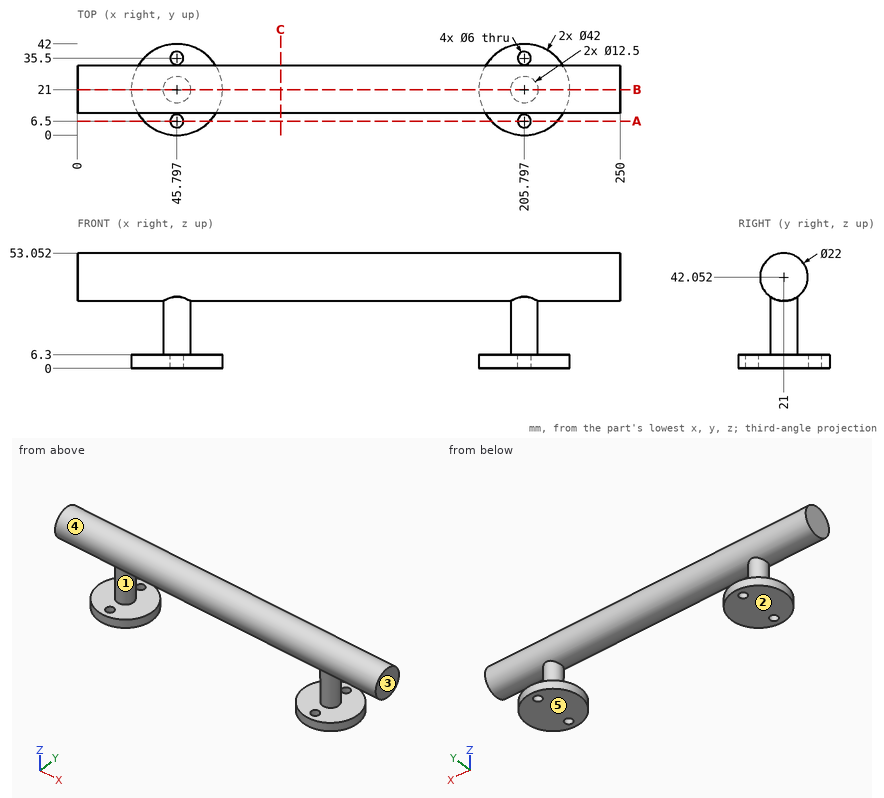
Geometry: see drawing. Coordinates: mm, zero at the bounding-box minimum. A direction names the side the tool comes from. Round coordinates to 2 decimals unless told otherwise and drop trailing zeros. Loops run counter-clockwise (first coordinate to the right, second up) from the corner with the lowest first, then second, coordinate; pieces in that order, holes last. Notation, with made-up numbers: (-25, -21) - (-1, -21) arc R18 ccw to (-1, -15) - close; hole circle Ø5 at (1, 27.5). An arc over 180 degrees is marked (long way). Write item = value, one per line. Start each with the question number.
(1) Set-up query: the marked faces 4 and 5. Return all of +Z, -Z, +X, -X, +Y, -Y with unobstructed straight access to the full face (end or side cutting, diameter ignored); none if empty.
(2) Section query A-A, the plane y = 6.5. Output: boundary loops of the cut face in (x, z).
(3) Section query B-B, the plane y = 21. Output: boundary loops of the cut face in (x, z).
(4) Pull-direction query (X, two-part tool) for the marked faces 1, 2 and 3; classes: +X half, -X half, draft (parallel to the pull), parting line (faces both ways), or undercut.
(5) Pin query (flat end, axial travel): pin 1 (4 mm diameter, centred on x = 204, y = 14, fed in from +Z); pin 2 (1 mm diameter, centred on x = 35.5, z = 36.5, fed in from +Y); pin 3 (5 mm diameter, centred on x = 80, z = 33, fed in from -Y) (1 decimal); pin 4 (8 mm diameter, centred on y = 14, z = 30.5, fed in from -X). Return the tip coordinate at first contact, or that it passes through.
(6) Section query C-C, the plane x = 93.5. Output: boundary loops of the cut face in (y, z), plus the area to 3 significant figures.
(7) Ray query, line 1 along X through (y, z) = (20.5, 22); line 2 along Y through (x, z) = (45, 3.5) (1 decimal); line 3 along Z through (x, y) = (56, 6). Return the intervals inside material, ascending. Write a range as from..to.
Conclusion:
q1.face_4 = none
q1.face_5 = -Z, +X, -X, +Y, -Y
q2.outline = (30.61, 0) - (42.8, 0) - (42.8, 6.3) - (30.61, 6.3) - close; (48.8, 0) - (60.99, 0) - (60.99, 6.3) - (48.8, 6.3) - close; (190.61, 0) - (202.8, 0) - (202.8, 6.3) - (190.61, 6.3) - close; (208.8, 0) - (220.99, 0) - (220.99, 6.3) - (208.8, 6.3) - close
q3.outline = (0, 31.05) - (39.55, 31.05) - (39.55, 6.3) - (24.8, 6.3) - (24.8, 0) - (66.8, 0) - (66.8, 6.3) - (52.05, 6.3) - (52.05, 31.05) - (199.55, 31.05) - (199.55, 6.3) - (184.8, 6.3) - (184.8, 0) - (226.8, 0) - (226.8, 6.3) - (212.05, 6.3) - (212.05, 31.05) - (250, 31.05) - (250, 53.05) - (0, 53.05) - close
q4.face_1 = undercut
q4.face_2 = draft
q4.face_3 = +X half
q5.pin_1 = 51.85
q5.pin_2 = 30.77
q5.pin_3 = 12.2
q5.pin_4 = 0
q6.outline = circle Ø22 at (21, 42.05)
q6.area = 380 mm2
q7.line_1 = 39.57..52.03, 199.57..212.03
q7.line_2 = 0..3.6, 9.4..32.6, 38.4..42
q7.line_3 = 0..6.3
